```python
from build123d import *

# Parameters (mm, degrees)
BOSS_EXTRUDE1_DEPTH     = 6.35
F_1_4_CLEARANCE_HOLE1_D = 6.7564
CUT_EXTRUDE1_DEPTH      = 679.542476995
SKETCH9_R               = 1.905
CUT_EXTRUDE2_DEPTH      = 679.542476995
BOSS_EXTRUDE2_DEPTH     = 6.35
FILLET1_R               = 2.54
FILLET2_R               = 7.62


with BuildPart() as part:
    # Sketch4 → Boss-Extrude1 (new body)
    with BuildSketch(Plane(origin=(0, 0, 0), x_dir=(0, 0, -1), z_dir=(1, 0, 0))):
        with BuildLine():
            Line((31.75, -280.9875), (76.2, -280.9875))
            Line((76.2, -280.9875), (76.2, -673.1))
            Line((76.2, -673.1), (31.75, -673.1))
            Line((31.75, -673.1), (15.282303513, -673.1))
            Line((15.282303513, -673.1), (-78.562742141, -332.832245873))
            ThreePointArc((-78.562742141, -332.832245873), (-85.532748147, -281.837746657), (-78.825143864, -230.808069226))
            Line((-78.825143864, -230.808069226), (-16.444584614, 0))
            Line((-16.444584614, 0), (0, 0))
            Line((0, 0), (73.025, 0))
            Line((73.025, 0), (73.025, -234.95))
            Line((73.025, -234.95), (31.75, -234.95))
            Line((31.75, -234.95), (31.75, -280.9875))
        make_face()
        with BuildLine():
            Line((-28.901727688, -92.33360131), (-10.677232282, -24.902968307))
            ThreePointArc((-10.677232282, -24.902968307), (-8.341183326, -23.560982736), (-6.999197755, -25.897031693))
            Line((-6.999197755, -25.897031693), (-25.223693161, -93.327664696))
            ThreePointArc((-25.223693161, -93.327664696), (-27.559742118, -94.669650267), (-28.901727688, -92.33360131))
        make_face(mode=Mode.SUBTRACT)
        with BuildLine():
            Line((-42.977227606, -416.480766903), (-61.548336892, -349.144770587))
            ThreePointArc((-61.548336892, -349.144770587), (-60.218385428, -346.801849525), (-57.875464366, -348.13180099))
            Line((-57.875464366, -348.13180099), (-39.304355079, -415.467797306))
            ThreePointArc((-39.304355079, -415.467797306), (-40.634306544, -417.810718368), (-42.977227606, -416.480766903))
        make_face(mode=Mode.SUBTRACT)
        with BuildLine():
            Line((7.967559467, -586.868515201), (-10.603549819, -519.532518885))
            ThreePointArc((-10.603549819, -519.532518885), (-12.946470881, -518.202567421), (-14.276422345, -520.545488483))
            Line((-14.276422345, -520.545488483), (4.294686941, -587.881484799))
            ThreePointArc((4.294686941, -587.881484799), (6.637608003, -589.211436263), (7.967559467, -586.868515201))
        make_face(mode=Mode.SUBTRACT)
        with BuildLine():
            Line((-58.723629262, -202.674637133), (-40.499133856, -135.24400413))
            ThreePointArc((-40.499133856, -135.24400413), (-38.163084899, -133.902018559), (-36.821099329, -136.238067516))
            Line((-36.821099329, -136.238067516), (-55.045594735, -203.668700519))
            ThreePointArc((-55.045594735, -203.668700519), (-57.381643691, -205.01068609), (-58.723629262, -202.674637133))
        make_face(mode=Mode.SUBTRACT)
    extrude(amount=BOSS_EXTRUDE1_DEPTH)

    # 1/4 Clearance Hole1 (through all)
    with Locations(Plane(origin=(6.35, 0, 0), x_dir=(0, 0, -1), z_dir=(1, 0, 0))):
        with Locations((53.975, -631.825), (53.975, -193.675), (48.181629833, -174.671224416), (38.787102693, -173.100083168), (56.593370167, -66.628775584)):
            Hole(F_1_4_CLEARANCE_HOLE1_D / 2)

    # Sketch7 → Cut-Extrude1 (cut, through all)
    with BuildSketch(Plane(origin=(6.35, 0, 0), x_dir=(0, 0, -1), z_dir=(1, 0, 0))):
        with BuildLine():
            Line((73.025, -72.801919324), (65.430665878, -71.531842458))
            ThreePointArc((65.430665878, -71.531842458), (62.655971682, -67.642685403), (66.545128736, -64.867991206))
            Line((66.545128736, -64.867991206), (73.025, -65.951685241))
            Line((73.025, -65.951685241), (73.025, -72.801919324))
        make_face()
    extrude(amount=-CUT_EXTRUDE1_DEPTH, mode=Mode.SUBTRACT)

    # Sketch9 → Cut-Extrude2 (cut, through all)
    with BuildSketch(Plane(origin=(6.35, 0, 0), x_dir=(0, 0, -1), z_dir=(1, 0, 0))):
        with Locations((33.655, -234.95)):
            Circle(SKETCH9_R)
        with Locations((33.655, -280.9875)):
            Circle(SKETCH9_R)
    extrude(amount=-CUT_EXTRUDE2_DEPTH, mode=Mode.SUBTRACT)

    # Sketch10 → Boss-Extrude2 (add)
    with BuildSketch(Plane(origin=(6.35, 0, 0), x_dir=(0, 0, -1), z_dir=(1, 0, 0))):
        Polygon((0, 0), (0, 22.225), (-10.437827857, 22.225), (-16.444584614, 0), align=None)
    extrude(amount=-BOSS_EXTRUDE2_DEPTH)

    # Fillet1
    fillet1_edges = [part.edges().sort_by_distance(p)[0] for p in [
        (3.175, -65.951685241, -73.025),
        (3.175, -72.801919324, -73.025),
        (3.175, -280.9875, -35.56),
        (3.175, -234.95, -35.56),
        (3.175, 22.225, 10.437827857),
        (3.175, 22.225, 0),
        (3.175, -280.9875, -76.2),
        (3.175, -673.1, -76.2),
        (3.175, -673.1, -15.282303513),
        (3.175, 0, -73.025),
        (3.175, -234.95, -73.025),
    ]]
    fillet(fillet1_edges, radius=FILLET1_R)

    # Fillet2
    fillet2_edges = [part.edges().sort_by_distance(p)[0] for p in [
        (3.175, 0, 0),
    ]]
    fillet(fillet2_edges, radius=FILLET2_R)


solid = part.part
```
Design review of the part built by this model. Coordinates are the model's own, in mm. A direction names the side the tool comes from. Give positions to 0.01 mm unless a question says otherwise; leave off trailing zeros. Order: outer loops, then holes, each group sorted by start corner. A loop starts at its lowest first (then second) coordinate and runs counter-clockwise, first axis right, second up. Notation, with made-up numbers: M 28,38 L 73,38 A29 ccw 73,74 Z; hole C 89,75 d11. An arc over 180 degrees is marked long. One line per question, with ' | ' between items. Start each with the question number.
Q1. We need section A-A (y = -156.5). Write out the cut boundary in (x, z) (3 decimals).
Q2. The part is to be moulded in two halves that separate along Y. For faces 3 (the face through (3.131, -59.09, 19.917)), 4 (the face through (0, -321, -12)), 5 (the face through (3.131, -504.403, 31.244)), 6 (the face through (3.13, -169.43, 49.74)), say which applies: +Y half, -Y half, draft (parallel to the pull), parting line (faces both ways), or undercut.
Q3. We need section B-B (x = 3.75). State how many separate pieces and enclosed holes the cut face has, plus the area to 3 significant figures.
Q4. We need section C-C (y = -266.5). Write out the cut boundary in (x, z).
Q5. For L1, parallel to Y at x = 1, z = -41; L2, parallel to Y at x = 0.5, z = -62.5; L3, parallel to Y at x = 4.5, z = -30.5, list the stretches that pass through material, from the lowest coordinate up. Write a range as [from, to].
Q6. Machinability: for faces 1 (the face through (6.35, -321, -12)), 2 (the face through (3.13, -553.74, 5.12)), which of the approach directions +Z, -Z, +X, -X, +Y, -Y give a long, thin tool a straight path to every point of the face, cutting with its end or side? Answer none if there is none.
Q7. For pin 1 Ø1.9 at (x, y) = (4, 11) entering from -Z; pin 2 Ø5.5 at (y, z) = (-66.63, -56.59) entering from +X; pin 3 Ø1.9 at (x, y) = (4, -42) entering from -Z (3 decimals); pin 4 Ø1 at (x, y) = (1.5, -440.5) entering from +Z, all flat-tipped, find the tip position at first contact; note any pin that passes through.
Returned:
1) outline: M 0,-73.025 L 6.35,-73.025 L 6.35,42.297 L 0,42.297 Z; M 0,46.244 L 6.35,46.244 L 6.35,58.742 L 0,58.742 Z
2) face 3: undercut | face 4: draft | face 5: -Y half | face 6: undercut
3) separate pieces: 1 | enclosed holes: 9 | area: 77,700 mm2
4) outline: M 0,-31.75 L 6.35,-31.75 L 6.35,84.96 L 0,84.96 Z
5) L1: [-673.1, -280.99], [-234.95, -175.65], [-170.55, 0] | L2: [-673.1, -280.99], [-234.95, 0] | L3: [-673.1, 0]
6) face 1: +Z, -Z, +X, +Y, -Y | face 2: +X, -X
7) pin 1: z = 0 | pin 2: through | pin 3: z = -73.025 | pin 4: z = 49.01
